Check sheet for the modelled part. Datum: model origin and axes. Units: mm. A direction names the side the tool comes from. Give positions to 0.01 mm unless a question says otherwise; leave off trailing zeros. Order: outer loops, then holes, each group sorted by start corner. A loop starts at its lowest first (then second) coordinate and runs counter-clockwise, first axis right, second up.
```python
from build123d import *

# Parameters (mm, degrees)
SKETCH037_W     = 72.5
SKETCH037_H     = 55
PAD018_DEPTH    = 60
SKETCH038_W     = 67.5
SKETCH038_H     = 50
POCKET013_DEPTH = 60.001
SKETCH039_W     = 67.5
SKETCH039_H     = 4
PAD019_DEPTH    = 50
SKETCH040_R     = 2.2
HOLE006_DEPTH   = 25
SKETCH041_W     = 28
SKETCH041_H     = 43
POCKET014_DEPTH = 4
SKETCH042_W     = 33
SKETCH042_H     = 50
SKETCH042_W_2   = 28
SKETCH042_H_2   = 43
PAD020_DEPTH    = 40
SKETCH043_W     = 20
SKETCH043_H     = 2
PAD021_DEPTH    = 43


with BuildPart() as part:
    # Sketch037 → Pad018 (new body)
    with BuildSketch(Plane.YZ.offset(120)):
        with Locations((1.26, 27.5)):
            Rectangle(SKETCH037_W, SKETCH037_H)
    extrude(amount=PAD018_DEPTH)

    # Sketch038 (on Face5 of Pad018) → Pocket013 (cut, through all)
    with BuildSketch(Plane(origin=(120, 0, 0), x_dir=(0, 1, 0), z_dir=(-1, 0, 0))):
        with Locations((1.25, -27.5)):
            Rectangle(SKETCH038_W, SKETCH038_H)
    extrude(amount=-POCKET013_DEPTH, mode=Mode.SUBTRACT)

    # Sketch039 (on Face8 of Pocket013) → Pad019 (join)
    with BuildSketch(Plane(origin=(0, 0, 2.5), x_dir=(0, -1, 0), z_dir=(0, 0, 1))):
        with Locations((-1.25, 130)):
            Rectangle(SKETCH039_W, SKETCH039_H)
    extrude(amount=PAD019_DEPTH)

    # Sketch040 (on Face16 of Pad019) → Hole006 (cut)
    with BuildSketch(Plane.YZ.offset(132)):
        with Locations((-25.99, 42.5)):
            Circle(SKETCH040_R)
        with Locations((-23, 9)):
            Circle(SKETCH040_R)
        with Locations((23, 9)):
            Circle(SKETCH040_R)
    extrude(amount=-HOLE006_DEPTH, mode=Mode.SUBTRACT)

    # Sketch041 (on Face16 of Hole006) → Pocket014 (cut)
    with BuildSketch(Plane.YZ.offset(132)):
        with Locations((0, 27.5)):
            Rectangle(SKETCH041_W, SKETCH041_H)
    extrude(amount=-POCKET014_DEPTH, mode=Mode.SUBTRACT)

    # Sketch042 (on Face16 of Pocket014) → Pad020 (join)
    with BuildSketch(Plane.YZ.offset(132)):
        with Locations((0, 27.5)):
            Rectangle(SKETCH042_W, SKETCH042_H)
        with Locations((0, 27.5)):
            Rectangle(SKETCH042_W_2, SKETCH042_H_2, mode=Mode.SUBTRACT)
    extrude(amount=PAD020_DEPTH)

    # Sketch043 (on Face29 of Pad020) → Pad021 (join)
    with BuildSketch(Plane(origin=(0, 0, 6), x_dir=(0, -1, 0), z_dir=(0, 0, 1))):
        with Locations((-4, 168.5)):
            Rectangle(SKETCH043_W, SKETCH043_H)
        with Locations((4, 157.333333)):
            Rectangle(SKETCH043_W, SKETCH043_H)
        with Locations((-4, 146.166667)):
            Rectangle(SKETCH043_W, SKETCH043_H)
        with Locations((4, 135)):
            Rectangle(SKETCH043_W, SKETCH043_H)
    extrude(amount=PAD021_DEPTH)


solid = part.part
```
(1) Cross-section at D-D on x = 131. Enter the section's corners in (y, z).
Response values:
outline: (-34.99, 0) - (37.51, 0) - (37.51, 55) - (-34.99, 55) - close; hole circle Ø4.4 at (-25.99, 42.5); hole circle Ø4.4 at (-23, 9); hole (-14, 6) - (14, 6) - (14, 49) - (-14, 49) - close; hole circle Ø4.4 at (23, 9)
(2) Material ranges on L1, parallel to Y at x = 147, z = 37; L2, parallel to X at y = -4, z = 37; L3, parallel to Y at x = 156, z = 5, recorded low to high.
Response values:
L1: y = -34.99 to -32.5, -16.5 to -14, -6 to 16.5, 35 to 37.51
L2: x = 134 to 136, 145.17 to 147.17, 156.33 to 158.33, 167.5 to 169.5
L3: y = -34.99 to -32.5, -16.5 to 16.5, 35 to 37.51
(3) Cross-section at A-A on x = 124. Enter the section's corners in (y, z).
Response values:
outline: (-34.99, 0) - (37.51, 0) - (37.51, 55) - (-34.99, 55) - close; hole (-32.5, 2.5) - (35, 2.5) - (35, 52.5) - (-32.5, 52.5) - close
(4) Cross-section at B-B on y = 23. Enter the section's corners in (x, z).
Response values:
outline: (120, 0) - (180, 0) - (180, 2.5) - (132, 2.5) - (132, 6.8) - (128, 6.8) - (128, 2.5) - (120, 2.5) - close; (120, 52.5) - (128, 52.5) - (128, 11.2) - (132, 11.2) - (132, 52.5) - (180, 52.5) - (180, 55) - (120, 55) - close
(5) Set-up check for faces 5 (the face through (124, 1, 2.5)), 6 (the face through (167.5, 4, 27)), 7 (the face through (130.03, -20.9, 9.66)), 8 (the face through (156, -32.5, 28)): record each of +Z, -Z, +X, -X, +Y, -Y from which the full face is reachable in a straight line by a thin tool's end or side.
Response values:
face 5: -X
face 6: none
face 7: +X, -X
face 8: +X
(6) Gauge pin test, flat ends, axial feed: pin 1 Ø5.5 at (y, z) = (23, 9) entering from +X; pin 2 Ø5 at (y, z) = (-2.5, 12.5) entering from +X; pin 3 Ø16 at (y, z) = (3, 37) entering from -X; pin 4 Ø14 at (x, y) = (142.5, -6.5) entering from -Z. Record the tip position at first contact, or that the pin passes through.
Response values:
pin 1: stops at x = 132
pin 2: stops at x = 169.5
pin 3: stops at x = 134
pin 4: stops at z = 0
(7) Cross-section at C-C on y = 7. Enter the section's corners in (x, z), then the cut area to 3 significant figures.
Response values:
outline: (120, 0) - (180, 0) - (180, 2.5) - (172, 2.5) - (172, 6) - (169.5, 6) - (169.5, 49) - (172, 49) - (172, 52.5) - (180, 52.5) - (180, 55) - (120, 55) - (120, 52.5) - (128, 52.5) - (128, 49) - (145.17, 49) - (145.17, 6) - (128, 6) - (128, 2.5) - (120, 2.5) - close; hole (147.17, 6) - (167.5, 6) - (167.5, 49) - (147.17, 49) - close
area: 780 mm2
(8) Release check for a two-part mould opening along Y. For faces 1 (the face through (150, 37.51, 27)), 2 (the face through (150, -34.99, 27)), 3 (the face through (150, 0, 6)), 4 (the face through (150, 1, 0)) record: released by +Y, released by -Y, zero draft, split by the parting line, or undercut.
Response values:
face 1: released by +Y
face 2: released by -Y
face 3: undercut
face 4: zero draft
